from build123d import *

# Parameters (mm, degrees)
SKETCH1_R                = 25
SKETCH1_R_2              = 11
BOSS_EXTRUDE1_DEPTH      = 10
CUT_EXTRUDE1_DEPTH       = 10
SKETCH5_R                = 1.75
CUT_EXTRUDE4_DEPTH       = 28.5
CUT_EXTRUDE4_DEPTH_BACK  = 23.5
CUT_EXTRUDE5_START       = 30
SKETCH6_R                = 3.5
CUT_EXTRUDE5_DEPTH       = 20
CUT_EXTRUDE6_START       = -30
CUT_EXTRUDE6_DEPTH       = 25
CUT_EXTRUDE8_START       = 20
CUT_EXTRUDE8_DEPTH       = 15
SKETCH9_W                = 20
SKETCH9_H                = 19.995459106
SKETCH9_R                = 1.75
BOSS_EXTRUDE2_DEPTH      = 10
CUT_EXTRUDE10_START      = 20
CUT_EXTRUDE10_DEPTH      = 1
CUT_EXTRUDE10_DEPTH_BACK = 17
SKETCH13_R               = 3.5
CUT_EXTRUDE11_DEPTH      = 5


with BuildPart() as part:
    # Sketch1 → Boss-Extrude1 (new body)
    with BuildSketch(Plane.XY):
        Circle(SKETCH1_R)
        Circle(SKETCH1_R_2, mode=Mode.SUBTRACT)
    extrude(amount=BOSS_EXTRUDE1_DEPTH)

    # Sketch2 → Cut-Extrude1 (cut)
    with BuildSketch(Plane.XY.offset(10)):
        Polygon((25, 0), (25, 2.5), (0, 2.5), (0, 0), (0, -2.5), (25, -2.5), align=None)
    extrude(amount=-CUT_EXTRUDE1_DEPTH, mode=Mode.SUBTRACT)

    # Sketch5 → Cut-Extrude4 (cut, two sides)
    with BuildSketch(Plane(origin=(0, -2.5, 0), x_dir=(1, 0, 0), z_dir=(0, 1, 0))) as cut_extrude4_sk:
        with Locations((17, -5)):
            Circle(SKETCH5_R)
    extrude(amount=CUT_EXTRUDE4_DEPTH, mode=Mode.SUBTRACT)
    extrude(cut_extrude4_sk.sketch, amount=-CUT_EXTRUDE4_DEPTH_BACK, mode=Mode.SUBTRACT)

    # Sketch6 → Cut-Extrude5 (cut)
    with BuildSketch(Plane(origin=(0, -2.5, 0), x_dir=(1, 0, 0), z_dir=(0, 1, 0)).offset(CUT_EXTRUDE5_START)):
        with Locations((17, -5)):
            Circle(SKETCH6_R)
    extrude(amount=-CUT_EXTRUDE5_DEPTH, mode=Mode.SUBTRACT)

    # Sketch7 → Cut-Extrude6 (cut)
    with BuildSketch(Plane(origin=(0, -2.5, 0), x_dir=(1, 0, 0), z_dir=(0, 1, 0)).offset(CUT_EXTRUDE6_START)):
        Polygon((21.041451884, -5), (19.020725942, -1.5), (14.979274058, -1.5), (12.958548116, -5), (14.979274058, -8.5), (19.020725942, -8.5), align=None)
    extrude(amount=CUT_EXTRUDE6_DEPTH, mode=Mode.SUBTRACT)

    # Sketch8 → Cut-Extrude8 (cut)
    with BuildSketch(Plane.XZ.offset(7.5).offset(CUT_EXTRUDE8_START)):
        Polygon((12.866790083, 5), (12.866790083, -1.917841475), (27.200285801, -1.917841475), (26.866413077, 13.440303847), (13.08223917, 14.012657089), (12.866790083, 14.617290025), align=None)
    extrude(amount=-CUT_EXTRUDE8_DEPTH, mode=Mode.SUBTRACT)

    # Sketch9 → Boss-Extrude2 (add)
    with BuildSketch(Plane(origin=(0, 0, 0), x_dir=(-1, 0, 0), z_dir=(0, 0, -1))):
        with Locations((32.913869245, 0)):
            Rectangle(SKETCH9_W, SKETCH9_H)
        with Locations((32.913869245, 5)):
            Circle(SKETCH9_R, mode=Mode.SUBTRACT)
        with Locations((32.913869245, -5)):
            Circle(SKETCH9_R, mode=Mode.SUBTRACT)
    extrude(amount=-BOSS_EXTRUDE2_DEPTH)

    # Sketch12 → Cut-Extrude10 (cut, two sides)
    with BuildSketch(Plane(origin=(0, 7.5, 0), x_dir=(1, 0, 0), z_dir=(0, 1, 0)).offset(CUT_EXTRUDE10_START)) as cut_extrude10_sk:
        Polygon((13.5, -5), (13.5, -13.927186896), (27.549462707, -13.927186896), (27.549462707, 2.179730433), (13.5, 2.179730433), align=None)
    extrude(amount=CUT_EXTRUDE10_DEPTH, mode=Mode.SUBTRACT)
    extrude(cut_extrude10_sk.sketch, amount=-CUT_EXTRUDE10_DEPTH_BACK, mode=Mode.SUBTRACT)

    # Sketch13 → Cut-Extrude11 (cut)
    with BuildSketch(Plane(origin=(0, 0, 0), x_dir=(-1, 0, 0), z_dir=(0, 0, -1))):
        with Locations((32.913869245, 5)):
            Circle(SKETCH13_R)
        with Locations((32.913869245, -5)):
            Circle(SKETCH13_R)
    extrude(amount=-CUT_EXTRUDE11_DEPTH, mode=Mode.SUBTRACT)


solid = part.part
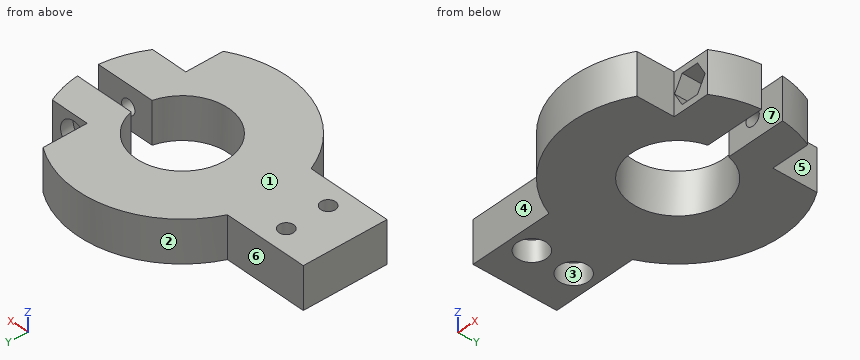
Build history of the part. All positions in model axes, mm. Face numbers are marked on the shaded views. A direction names the side the tool comes from. Round coordinates to 2 decimals unless told otherwise and drop trailing zeros. Loops run counter-clockwise (first coordinate to the right, second up) from the corner with the lowest first, then second, coordinate; pieces in that order, holes last. Notation, with made-up numbers: (2, 53.5) -> (16, 53.5) arc R34 ccw to (16, 91.5) -> close; hole circle Ø6 at (38, -38). An arc over 180 degrees is marked (long way). One line per item, written item: value. Start each with the question number.
Q1. Drop flat-ended pins along their axis: pin 1 Ø5 at (x, z) = (-22, 5) entering from -Y; pin 2 Ø2 at (y, z) = (13.5, 8) entering from +X; pin 3 Ø2 at (x, z) = (16, 5) entering from +Y. Give the stop position or say it passes through.
Q2. Probe line 1 along Y through (x, z) = (0, 7.25); line 2 along X through (y, z) = (6, 3.75); line 3 along Y through (x, z) = (16.5, 9). List the from-to ranges inside material, lowest first.
Q3. 3-axis set-ups, long thin cutter, end or side, ignore diameter. For the marked faces 5, 6 and 7: which of +Z, -Z, +X, -X, +Y, -Y reach the whole face in a straight line?
Q4. Cut at C-C on z = 7.75. List the corners of the cut face in (x, y), plus the area to 3 significant figures.
Q5. Cut at A-A on x = 0. List the corners of the cut face in (y, z).
Q6. Cut at B-B on y = 5. List the corners of the cut face in (x, z).
Q7. Cut at D-D on y = 0. List the corners of the cut face in (x, z).
Q8. Two-plate mould, pull along Y, no slides. Class the marked faces 1, 2, 3 and 4: released by +Y, released by -Y, zero draft, split by the parting line, or undercut.
Computed:
1. pin 1: y = -15.64
1. pin 2: x = 13.5
1. pin 3: y = 7.5
2. line 1: -25 to -11, 11 to 25
2. line 2: -42.91 to -36.27, -29.56 to -9.22, 9.22 to 15.78, 18.22 to 24.27
2. line 3: -12.5 to -2.5, 2.5 to 10.5
3. face 5: +Z, -Z, +X, +Y
3. face 6: +Z, -Z, -X, +Y
3. face 7: +Z, -Z, +X
4. outline: (-42.91, -10) -> (-22.91, -10) arc R25 ccw to (12.87, -21.43) -> (12.87, -12.5) -> (14.55, -12.5) -> (14.55, -7.5) -> (19.45, -7.5) -> (19.45, -12.5) -> (21.65, -12.5) arc R25 ccw to (24.87, -2.5) -> (10.71, -2.5) arc R11 cw (long way) to (10.71, 2.5) -> (24.87, 2.5) arc R25 ccw to (22.69, 10.5) -> (19.17, 10.5) -> (19.17, 7.5) -> (14.83, 7.5) -> (14.83, 10.5) -> (13.5, 10.5) -> (13.5, 21.04) arc R25 ccw to (-22.91, 10) -> (-42.91, 10) -> close; hole circle Ø3.5 at (-32.91, -5); hole circle Ø3.5 at (-32.91, 5)
4. area: 1,720 mm²
5. outline: (-25, 0) -> (-11, 0) -> (-11, 10) -> (-25, 10) -> close; (11, 0) -> (25, 0) -> (25, 10) -> (11, 10) -> close
6. outline: (-42.91, 0) -> (-36.41, 0) -> (-36.41, 5) -> (-34.66, 5) -> (-34.66, 10) -> (-42.91, 10) -> close; (-31.16, 5) -> (-29.41, 5) -> (-29.41, 0) -> (-9.8, 0) -> (-9.8, 10) -> (-31.16, 10) -> close; (9.8, 0) -> (24.49, 0) -> (24.49, 10) -> (9.8, 10) -> close; hole circle Ø3.5 at (17, 5)
7. outline: (-42.91, 0) -> (-11, 0) -> (-11, 10) -> (-42.91, 10) -> close
8. face 1: zero draft
8. face 2: released by +Y
8. face 3: undercut
8. face 4: released by -Y
